Drawing for the job (mm, zero at the part's lowest x, y, z). A direction names the side the tool comes from. Give positions to 0.01 mm unless a question says otherwise; leave off trailing zeros. Write each loop counter-clockwise with the first axis right and the second up, starting at its lowest first coordinate (ties: lowest second). Pieces come first, ordered by that corner, then holes. Notation, with made-up numbers: M 53.25,47 L 86.25,47 A24 cw 86.25,73 Z; hole C -8.5,9.25 d10. An arc over 180 degrees is marked long. Use CSV: the item, a comma, the result in double quotes. Start each with the question number.
1. 3-axis set-ups, long thin cutter, end or side, ignore diameter. For the marked faces 1, 2 and 3: which of +Z, -Z, +X, -X, +Y, -Y reach the whole face in a straight line?
2. Band-saw the part on C-C, the plane x = 20. List the corners of the cut face in (y, z), then the cut area to 3 significant figures.
3. Drill centre lines: line 1 along X through (y, z) = (60, 0.75); line 2 along X through (y, z) = (38.5, 1); line 3 along Y through (x, z) = (186.5, 3.75). Where is each one in solid material? Low to high. Write a range as from..to.
4. Drop flat-ended pins along their axis: pin 1 Ø3 at (x, z) = (149.5, 7.5) entering from -Y; pin 2 Ø4 at (y, z) = (42.5, 8.5) entering from -X; pin 3 Ø6.5 at (y, z) = (57, 4.5) entering from -X; pin 4 Ø4 at (y, z) = (58.5, 7.5) entering from +X. Give the stop position or say it passes through.
5. Mould opens along X. For the marked faces 4, 5 and 6 say: pulls with the +X half, pulls with the -X half, needs draft (parallel to the pull), parting line crosses it, or undercut.
6. Band-saw the part on A-A, the plane z = 5.5. List the corners of the cut face in (x, y), then the cut area to 3 significant figures.
7. Band-saw the part on B-B, the plane y = 4. List the corners of the cut face in (x, z).
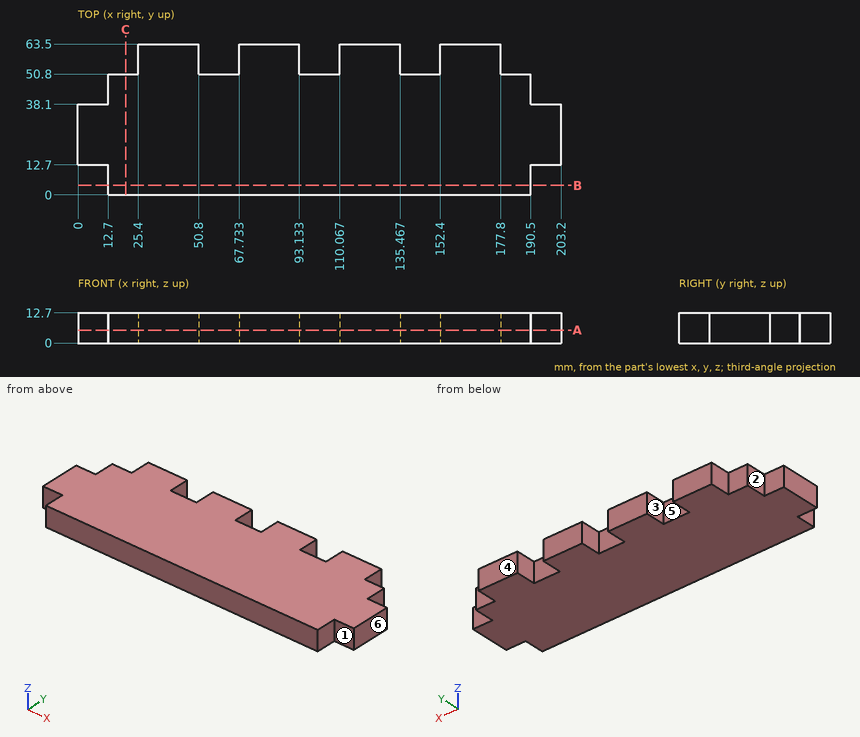
Output:
1,face 1,"+Z, -Z, +X, -Y"
1,face 2,"+Z, -Z, -X, +Y"
1,face 3,"+Z, -Z, +Y"
2,outline,"M 0,0 L 50.8,0 L 50.8,12.7 L 0,12.7 Z"
2,area,"645 mm²"
3,line 1,"x = 25.4..50.8, 67.73..93.13, 110.07..135.47, 152.4..177.8"
3,line 2,"x = 12.7..190.5"
3,line 3,"y = 0..50.8"
4,pin 1,"stops at y = 0"
4,pin 2,"stops at x = 12.7"
4,pin 3,"stops at x = 25.4"
4,pin 4,"stops at x = 177.8"
5,face 4,"needs draft"
5,face 5,"undercut"
5,face 6,"pulls with the +X half"
6,outline,"M 0,12.7 L 12.7,12.7 L 12.7,0 L 190.5,0 L 190.5,12.7 L 203.2,12.7 L 203.2,38.1 L 190.5,38.1 L 190.5,50.8 L 177.8,50.8 L 177.8,63.5 L 152.4,63.5 L 152.4,50.8 L 135.47,50.8 L 135.47,63.5 L 110.07,63.5 L 110.07,50.8 L 93.13,50.8 L 93.13,63.5 L 67.73,63.5 L 67.73,50.8 L 50.8,50.8 L 50.8,63.5 L 25.4,63.5 L 25.4,50.8 L 12.7,50.8 L 12.7,38.1 L 0,38.1 Z"
6,area,"11,000 mm²"
7,outline,"M 12.7,0 L 190.5,0 L 190.5,12.7 L 12.7,12.7 Z"
